The listing builds one solid part. Answer for the finished solid, in the listing's coordinates (mm). A direction names the side the tool comes from. Round coordinates to 2 decimals unless told otherwise and drop trailing zeros. Order: outer loops, then holes, each group sorted by start corner. A loop starts at its lowest first (then second) coordinate and runs counter-clockwise, first axis right, second up. Notation, with made-up numbers: M 14.25,70.5 L 45.25,70.5 A8 ccw 45.25,77.5 Z; hole C 38.25,43.25 d10. An arc over 180 degrees is marked long. Write item = value, one per line. Start each with the question number.
(1) A cutting plane is placed at B-B, the plane y = 35.5. Determine the outline of the cut face in (x, z) (3 decimals), and give its area (3 significant figures).
(2) For a pull along X with two mould halves and no side action, classify faces 1 (the face through (22.225, 17, 19)), 2 (the face through (-3, 7.938, 30)), 3 (the face through (59, 2, 42.875)), 4 (the face through (41.275, -1, 5)) as released by +X, released by -X, zero draft, split by the parting line, or undercut.
(3) Each of these flat-tipped pins is pushed along its axis until it touches: pin 1 (15.5 mm diameter, centred on x = 89, y = -4.5, fed in from -Z); pin 2 (4 mm diameter, centred on x = 94, z = 53.5, fed in from -Y); pin 3 (19 mm diameter, centred on y = -14.5, z = 20.5, fed in from -X). Where does it stop, or does it pass through?
(4) Which of the six approach directions +Z, -Z, +X, -X, +Y, -Y give full straight-line access (tool end or side, diameter ignored) to faces 5 (the face through (39.464, 61.59, 0.133)), 6 (the face through (59, -2, 61.925)), 7 (the face through (31.89, 16.55, 51.12)), 8 (the face through (45.898, -0.356, 38.202)), 9 (the face through (45, -25.4, 42))?
(5) Straight lines are drawn through the part: probe 1 along Z at (x, y) = (-30.5, 35) (3 decimals); probe 2 along Y at (x, z) = (-31, 15); probe 3 along Y at (x, z) = (44, 43). For each, find the intervals that lie inside material, in ascending order. Write a range as from..to.
(6) A cutting plane is placed at A-A, the plane z = -2. Determine the outline of the cut face in (x, y) (3 decimals).
from build123d import *

# Parameters (mm, degrees)
F1_DEPTH = 63.5
F2_DEPTH = 25.4
F3_DEPTH = 7.9375
F5_R     = 6.35


with BuildPart() as f1:
    # F0 (on Front) → F1 (new body, symmetric)
    with BuildSketch(Plane.XZ):
        Polygon((-41.275, -9.525), (41.275, -9.525), (41.275, 9.525), (22.225, 9.525), (-41.275, 9.525), align=None)
    extrude(amount=F1_DEPTH, both=True)

    # F0 (on Front) → F2 (join, symmetric)
    with BuildSketch(Plane.XZ):
        with BuildLine():
            Line((22.225, 9.525), (41.275, 9.525))
            Line((41.275, 9.525), (41.275, 27.277773))
            ThreePointArc((41.275, 27.277773), (46.020823, 38.323232), (57.147573, 42.8752))
            Line((57.147573, 42.8752), (60.325, 42.8752))
            Line((60.325, 42.8752), (60.325, 57.277))
            Line((60.325, 57.277), (60.325, 61.9252))
            Line((60.325, 61.9252), (57.147573, 61.9252))
            add(Edge.make_bspline(
                [(54.397042, 61.816722), (55.308689, 61.860952), (56.225552, 61.897181), (57.147573, 61.9252)],
                knots=[109.785705, 109.785705, 109.785705, 109.785705, 111.502394, 111.502394, 111.502394, 111.502394], degree=3))
            ThreePointArc((54.397042, 61.816722), (31.637999, 50.854282), (22.225, 27.411915))
            Line((22.225, 27.411915), (22.225, 9.525))
        make_face()
        Polygon((60.325, 57.277), (60.325, 42.8752), (85.450254, 42.8752), (85.450254, 61.9252), (60.325, 61.9252), align=None)
    extrude(amount=F2_DEPTH, both=True)

    # F0 (on Front) → F3 (join, symmetric)
    with BuildSketch(Plane.XZ):
        with BuildLine():
            add(Edge.make_bspline(
                [(-41.275, 9.525), (-40.874115, 23.43416), (-3.90464, 58.988111), (54.397042, 61.816722)],
                knots=[0, 0, 0, 0, 109.785705, 109.785705, 109.785705, 109.785705], degree=3))
            Line((-41.275, 9.525), (22.225, 9.525))
            Line((22.225, 9.525), (22.225, 27.411915))
            ThreePointArc((22.225, 27.411915), (31.637999, 50.854282), (54.397042, 61.816722))
        make_face()
    extrude(amount=F3_DEPTH, both=True)

    # F0 (on Front) → F4 (revolve)
    with BuildSketch(Plane.XZ):
        Polygon((85.450254, 61.9252), (85.450254, 42.8752), (85.725, 38.1), (111.125, 38.1), (111.125, 66.675), (85.725, 66.675), align=None)
    revolve(axis=Axis((85.450254, 0, 52.4002), (0, 0, -1)))

    # F5
    f5_edges = [f1.edges().sort_by_distance(p)[0] for p in [
        (41.275, -63.5, 0),
        (-41.275, -63.5, 0),
        (41.275, 63.5, 0),
        (-41.275, 63.5, 0),
    ]]
    fillet(f5_edges, radius=F5_R)


solid = f1.part
Reported:
q1.outline = M -41.275,-9.525 L 41.275,-9.525 L 41.275,9.525 L -41.275,9.525 Z
q1.area = 1,570 mm²
q2.face_1 = released by -X
q2.face_2 = zero draft
q2.face_3 = undercut
q2.face_4 = released by +X
q3.pin_1 = 38.1
q3.pin_2 = -24.83
q3.pin_3 = -40.34
q4.face_5 = +Z, -Z, +X, +Y
q4.face_6 = +Z, -X
q4.face_7 = +Z, -X, +Y
q4.face_8 = -Z, +Y, -Y
q4.face_9 = +Z, -X, -Y
q5.probe_1 = -9.525..9.525
q5.probe_2 = -7.94..7.94
q5.probe_3 = -25.4..25.4
q6.outline = M -41.275,-57.15 A6.35 ccw -34.925,-63.5 L 34.925,-63.5 A6.35 ccw 41.275,-57.15 L 41.275,57.15 A6.35 ccw 34.925,63.5 L -34.925,63.5 A6.35 ccw -41.275,57.15 Z
